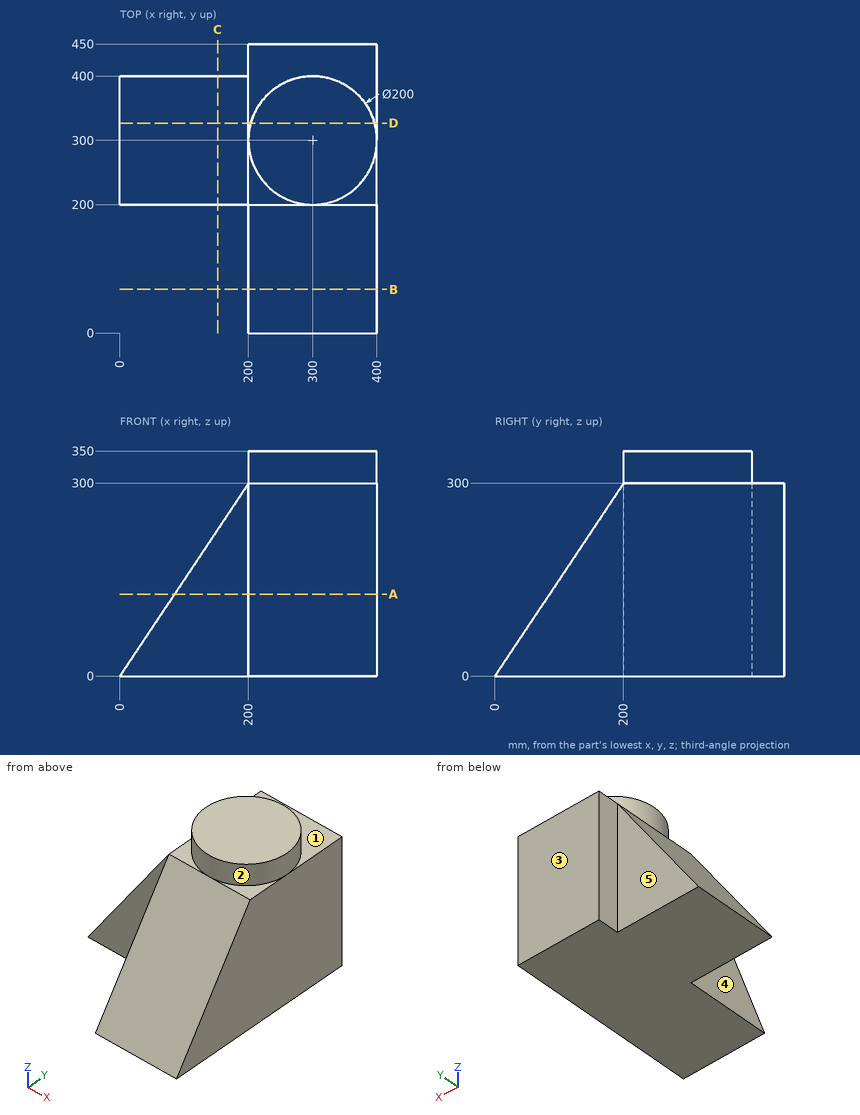
Job drawing, mm, ordinate dimensions from the low corner. One solid piece. A direction names the side the tool comes from. Coordinates: 2 decimals unless noted, no trailing zeros. Write each loop counter-clockwise with the first axis right and the second up, starting at its lowest first coordinate (ties: lowest second). Pieces come first, ordered by that corner, then holes. Notation, with made-up numbers: M 33.5,51.5 L 56.5,51.5 A16 ccw 56.5,60.5 Z; hole C -1.75,-10.5 d2. An arc over 180 degrees is marked long. Answer as a JSON object with one key per item and string values. Group by question number.
1) Saw through at B-B (y = 68). Write the cut outline in (x, z), plus the area to 3 significant figures.
2) Pin check, flat tips, straight feed: pin 1 Ø8 at (x, y) = (308, 193) entering from +Z; pin 2 Ø10 at (y, z) = (142, 218.5) entering from -X; pin 3 Ø8 at (x, y) = (154, 290.5) entering from +Z. Stop position of each tip, or through.
3) Wall check: line 1 (X direction, y = 163, z = 211); line 2 (Z direction, x = 225.5, y = 207). Give the ranges that are in metal, low to high. Write a range as from..to.
4) Saw through at D-D (y = 327). Write the cut outline in (x, z).
5) Saw through at C-C (x = 152). Write the cut outline in (y, z), plus the area to 3 significant figures.
6) Tool access for the marked faces 1, 2, 3, 4 and 5: list every direction of +Z, -Z, +X, -X, +Y, -Y with a clear straight run to the whole face (end or side of a thin tool).
7) Saw through at A-A (z = 127.5). Write the cut outline in (x, y).
Values follow:
{
 "1": {"outline": "M 200,0 L 400,0 L 400,102 L 200,102 Z", "area": "20,400 mm2"},
 "2": {"pin 1": "stops at z = 295.5", "pin 2": "stops at x = 200", "pin 3": "stops at z = 237"},
 "3": {"line 1": "x = 200..400", "line 2": "z = 0..300"},
 "4": {"outline": "M 0,0 L 400,0 L 400,300 L 396.29,300 L 396.29,350 L 203.71,350 L 203.71,300 L 200,300 Z"},
 "5": {"outline": "M 200,0 L 400,0 L 400,228 L 200,228 Z", "area": "45,600 mm2"},
 "6": {"face 1": "+Z, +Y", "face 2": "+Z", "face 3": "+Z, -Z, +X, -X, +Y", "face 4": "+Z, -Z, -X, -Y", "face 5": "+Z, -Z, -X, +Y"},
 "7": {"outline": "M 85,200 L 200,200 L 200,85 L 400,85 L 400,450 L 200,450 L 200,400 L 85,400 Z"}
}
